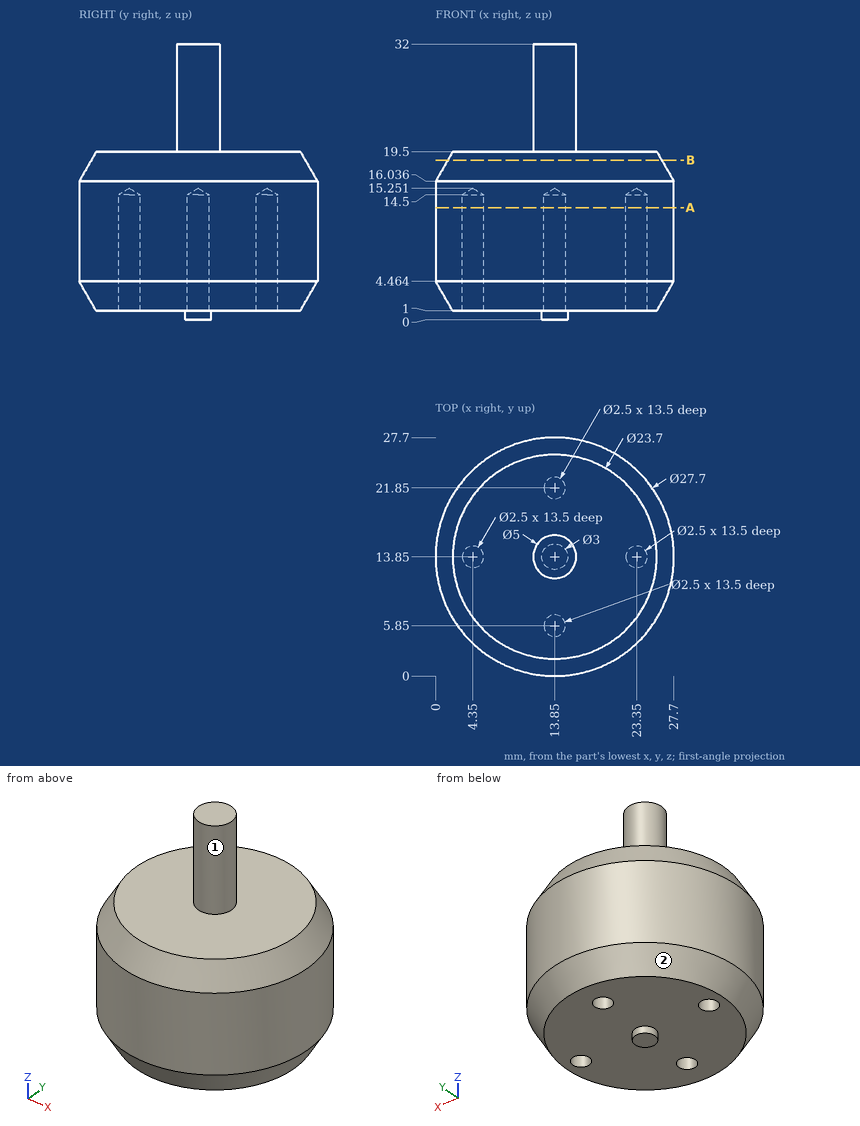
For this review, use the dimensioned drawing (mm, ordinates from the lowest corner) and the shaded views. A direction names the side the tool comes from. Coordinates: 2 decimals unless noted, no trailing zeros. Order: outer loops, then holes, each group sorted by start corner. A loop starts at its lowest first (then second) coordinate and runs counter-clockwise, first axis right, second up. Notation, with made-up numbers: (-19, 22.5) - (-3, 22.5) arc R18 cw to (-3, 38.5) - close; hole circle Ø10 at (36, 46). An arc over 180 degrees is marked (long way). Answer as a JSON object with one key per item and string values. Group by question number.
1. We need section B-B on z = 18.5. State the section outline as (x, y) points, then the cut area to 3 significant figures.
2. For probe 1 along Y at (x, z) = (13.85, 8.5); probe 2 along Z at (x, y) = (9.75, 3); probe 3 along Y at (x, z) = (4.25, 8.5), list the stretches that pass through material, from the lowest coordinate up.
3. For the marked faces 1 and 2, list the 3-axis set-ups (+Z, -Z, +X, -X, +Y, -Y) from which the entire face can be reached by the end or side of a thin tool; tool diameter is ignored.
4. We need section A-A on z = 13. State the section outline as (x, y) points.
5. Clearance check with flat-ended pins moving along their axes: P1, Ø8, axis at x = 14.5, y = 21.5, coming from the -Z side; P2, Ø3, axis at y = 21, z = 10.5, coming from the -X side (3 decimals); P3, Ø2, axis at x = 13.85, y = 21.85, coming from the -Z side. State where each tip first meets the part, or that it passes through.
Final values:
{
 "1": {"outline": "circle Ø24.85 at (13.85, 13.85)", "area": "485 mm²"},
 "2": {"probe 1": "0 to 4.6, 7.1 to 20.6, 23.1 to 27.7", "probe 2": "1 to 19.5", "probe 3": "3.87 to 12.6, 15.1 to 23.83"},
 "3": {"face 1": "+Z", "face 2": "-Z"},
 "4": {"outline": "circle Ø27.7 at (13.85, 13.85); hole circle Ø2.5 at (4.35, 13.85); hole circle Ø2.5 at (13.85, 5.85); hole circle Ø2.5 at (13.85, 21.85); hole circle Ø2.5 at (23.35, 13.85)"},
 "5": {"P1": "z = 1", "P2": "x = 1.205", "P3": "z = 14.65"}
}
